Read the model definition and answer for the solid it produces. Units are mm, in the model's axes. Face numbers are marked on the shaded views. A direction names the side the tool comes from. Coordinates: 2 decimals unless noted, no trailing zeros. Order: outer loops, then holes, each group sorted by start corner. A loop starts at its lowest first (then second) coordinate and runs counter-clockwise, first axis right, second up. Notation, with made-up numbers: M 70.25,46.5 L 125.25,46.5 A31 ccw 125.25,82.5 Z; hole C -24,10.5 d1. An arc over 180 degrees is marked long. Write each question's results on one line, items separated by ' | '.
```python
from build123d import *

# Parameters (mm, degrees)
SKETCH4_R           = 0.340929453
BOSS_EXTRUDE1_DEPTH = 4.7625


with BuildPart() as part:
    # Sketch3 → Revolve1 (revolve)
    with BuildSketch(Plane(origin=(0, 0, 0), x_dir=(1, 0, 0), z_dir=(0, 1, 0))):
        Polygon((0, 0), (0, 3.18516), (3.1623, 3.18516), (3.1623, 3.8354), (4.2799, 3.8354), (4.2799, 1.6129), (7.9629, 1.6129), (7.9629, 0), (4.318, 0), (4.318, -13.5128), (0, -13.5128), align=None)
    revolve(axis=Axis((0, 0, 13.5128), (0, 0, -1)))

    # Sketch4 → Boss-Extrude1 (add)
    with BuildSketch(Plane(origin=(0, 0, -3.18516), x_dir=(-1, 0, 0), z_dir=(0, 0, -1))):
        with Locations((0, 1.516184255)):
            Circle(SKETCH4_R)
        with Locations((1.313054082, -0.758092128)):
            Circle(SKETCH4_R)
        with Locations((-1.313054082, -0.758092128)):
            Circle(SKETCH4_R)
    extrude(amount=BOSS_EXTRUDE1_DEPTH)


solid = part.part
```
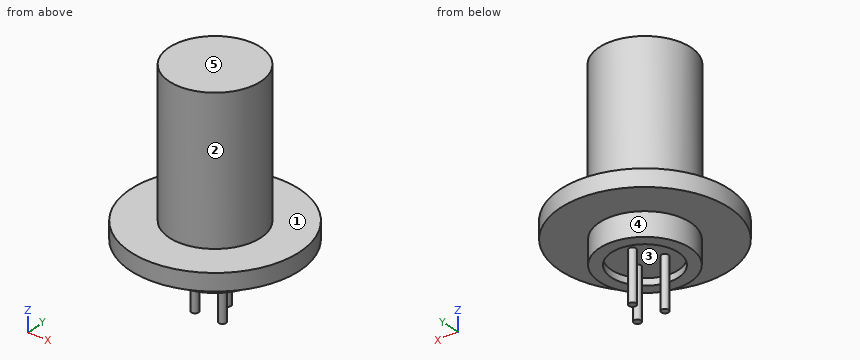
(1) The part is cut by section D-D, the plane x = -3.5. Write down the section's boundary in (y, z).
Conclusion:
outline: M -7.15,-1.61 L -2.46,-1.61 L -2.46,-3.84 L 2.46,-3.84 L 2.46,-1.61 L 7.15,-1.61 L 7.15,0 L 2.53,0 L 2.53,13.51 L -2.53,13.51 L -2.53,0 L -7.15,0 Z
(2) For the marked faces 4 and 5, determine the directions among +Z, -Z, +X, -X, +Y, -Y from which every point of the face is accessible in a straight line to the end or side of a thin tool.
Conclusion:
face 4: -Z | face 5: +Z, +X, -X, +Y, -Y
(3) Straight lines are drawn through the part: line 1 (Y direction, x = 0, z = -3.4); line 2 (X direction, y = 0, z = -3.5); line 3 (Z direction, x = -6.75, y = 2.5). For each, find the intervals that lie inside material, in ascending order.
Conclusion:
line 1: -4.28 to -3.16, 1.18 to 1.86, 3.16 to 4.28 | line 2: -4.28 to -3.16, 3.16 to 4.28 | line 3: -1.61 to 0
(4) The part is cut by section A-A, the plane y = 0. Write down the section's boundary in (x, z).
Conclusion:
outline: M -7.96,-1.61 L -4.28,-1.61 L -4.28,-3.84 L -3.16,-3.84 L -3.16,-3.19 L 3.16,-3.19 L 3.16,-3.84 L 4.28,-3.84 L 4.28,-1.61 L 7.96,-1.61 L 7.96,0 L 4.32,0 L 4.32,13.51 L -4.32,13.51 L -4.32,0 L -7.96,0 Z
(5) The mould has two halves that part along Y. Classify the marked faces 1, 2 and 3: pulls with the +Y half, pulls with the -Y half, needs draft (parallel to the pull), parting line crosses it, or undercut.
Conclusion:
face 1: needs draft | face 2: parting line crosses it | face 3: undercut
(6) The part is cut by section C-C, the plane z = 5.5. Write down the section's boundary in (x, y).
Conclusion:
outline: C 0,0 d8.64
(7) The part is cut by section B-B, the plane x = 0. Write down the section's boundary in (y, z), then the cut area to 3 significant figures.
Conclusion:
outline: M -7.96,-1.61 L -4.28,-1.61 L -4.28,-3.84 L -3.16,-3.84 L -3.16,-3.19 L 1.18,-3.19 L 1.18,-7.95 L 1.86,-7.95 L 1.86,-3.19 L 3.16,-3.19 L 3.16,-3.84 L 4.28,-3.84 L 4.28,-1.61 L 7.96,-1.61 L 7.96,0 L 4.32,0 L 4.32,13.51 L -4.32,13.51 L -4.32,0 L -7.96,0 Z | area: 161 mm²
(8) Given pin 1 (8 mm diameter, centred on y = 1.5, z = 5.5, fed in from +X); pin 2 (1.5 mm diameter, centred on x = -4.5, y = 3.5, fed in from +Z); pin 3 (1.5 mm diameter, centred on x = -2, z = 9.5, fed in from -Y), each flat-ended and moving along its own axis, determine where each tip first touches the part or whether it passes through.
Conclusion:
pin 1: x = 4.32 | pin 2: z = 0 | pin 3: y = -4.13
